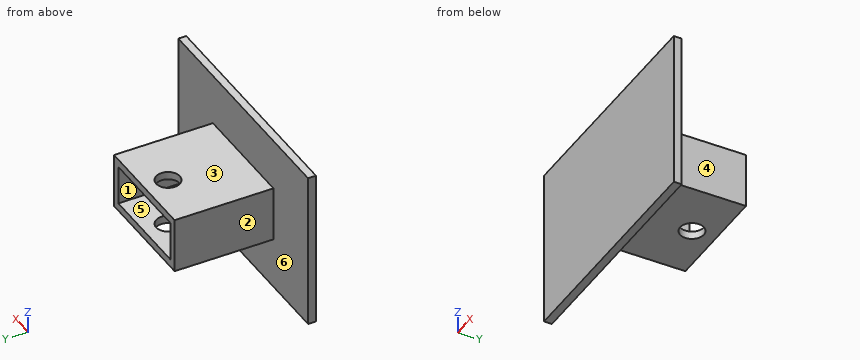
```python
from build123d import *

# Parameters (mm, degrees)
SKETCH1_W           = 76.2
SKETCH1_H           = 50.8
BOSS_EXTRUDE1_DEPTH = 2.54
SKETCH2_W           = 35.56
SKETCH2_H           = 17.78
SKETCH2_W_2         = 30.48
SKETCH2_H_2         = 12.7
BOSS_EXTRUDE2_DEPTH = 31.75
SKETCH3_R           = 3.81
CUT_EXTRUDE1_DEPTH  = 31.75


with BuildPart() as part:
    # Sketch1 → Boss-Extrude1 (new body)
    with BuildSketch(Plane(origin=(0, 0, 0), x_dir=(1, 0, 0), z_dir=(0, 1, 0))):
        Rectangle(SKETCH1_W, SKETCH1_H)
    extrude(amount=BOSS_EXTRUDE1_DEPTH)

    # Sketch2 → Boss-Extrude2 (add)
    with BuildSketch(Plane(origin=(0, 2.54, 0), x_dir=(1, 0, 0), z_dir=(0, 1, 0))):
        Rectangle(SKETCH2_W, SKETCH2_H)
        Rectangle(SKETCH2_W_2, SKETCH2_H_2, mode=Mode.SUBTRACT)
    extrude(amount=BOSS_EXTRUDE2_DEPTH)

    # Sketch3 → Cut-Extrude1 (cut)
    with BuildSketch(Plane.XY.offset(8.89)):
        with Locations((0, 26.67)):
            Circle(SKETCH3_R)
    extrude(amount=-CUT_EXTRUDE1_DEPTH, mode=Mode.SUBTRACT)


solid = part.part
```
For this review, take the finished solid that the model builds, in its own axes (mm). Face numbers are marked on the shaded views. A direction names the side the tool comes from. Give positions to 0.01 mm unless a question says otherwise; leave off trailing zeros. Write each loop counter-clockwise with the first axis right and the second up, starting at its lowest first coordinate (ties: lowest second). Pieces come first, ordered by that corner, then holes.
Item 1: Take a section at C-C (z = -1.5). Give the boundary of the cut face in (x, y), and give its area (3 significant figures).
Item 2: Wall thickness on probe 1 along Z at (x, y) = (-12, 22.5); probe 2 along X at (y, z) = (5, 5.5); probe 3 along Y at (x, z) = (0, 7.3): over which ranges is each line inside the solid? List them lowest first.
Item 3: Take a section at A-A (x = 0). Give the boundary of the cut face in (y, z).
Item 4: Insertion check: P1, Ø1.5, axis at x = 14.5, y = 16, coming from the -Z side; P2, Ø19.5, axis at y = 12.5, z = -0.5, coming from the -X side; P3, Ø10, axis at y = 21.5, z = -2, coming from the +X side. Each pin has a flat end and moves straight along its axis. Give the tip position at first contact, or say it passes through.
Item 5: Take a section at B-B (y = 26.67). Give the boundary of the cut face in (x, z).
Item 6: Take a section at D-D (x = -16.5). Give the boundary of the cut face in (y, z).
Item 7: Machinability: for the marked faces 1, 2 and 3, which of the approach directions +Z, -Z, +X, -X, +Y, -Y give a long, thin tool a straight path to every point of the face, cutting with its end or side? Answer none if there is none.
Item 8: The part is to be moulded in two halves that separate along X. For the marked faces 4, 5 and 6, say which applies: +X half, -X half, draft (parallel to the pull), parting line (faces both ways), or undercut.
Established:
1. outline: (-38.1, 0) - (38.1, 0) - (38.1, 2.54) - (17.78, 2.54) - (17.78, 34.29) - (15.24, 34.29) - (15.24, 2.54) - (-15.24, 2.54) - (-15.24, 34.29) - (-17.78, 34.29) - (-17.78, 2.54) - (-38.1, 2.54) - close
1. area: 355 mm2
2. probe 1: z = -8.89 to -6.35, 6.35 to 8.89
2. probe 2: x = -17.78 to -15.24, 15.24 to 17.78
2. probe 3: y = 0 to 22.86, 30.48 to 34.29
3. outline: (0, -25.4) - (2.54, -25.4) - (2.54, -8.89) - (22.86, -8.89) - (22.86, -6.35) - (2.54, -6.35) - (2.54, 6.35) - (22.86, 6.35) - (22.86, 8.89) - (2.54, 8.89) - (2.54, 25.4) - (0, 25.4) - close; (30.48, -8.89) - (34.29, -8.89) - (34.29, -6.35) - (30.48, -6.35) - close; (30.48, 6.35) - (34.29, 6.35) - (34.29, 8.89) - (30.48, 8.89) - close
4. P1: stops at z = -8.89
4. P2: stops at x = -17.78
4. P3: stops at x = 17.78
5. outline: (-17.78, -8.89) - (-3.81, -8.89) - (-3.81, -6.35) - (-15.24, -6.35) - (-15.24, 6.35) - (-3.81, 6.35) - (-3.81, 8.89) - (-17.78, 8.89) - close; (3.81, -8.89) - (17.78, -8.89) - (17.78, 8.89) - (3.81, 8.89) - (3.81, 6.35) - (15.24, 6.35) - (15.24, -6.35) - (3.81, -6.35) - close
6. outline: (0, -25.4) - (2.54, -25.4) - (2.54, -8.89) - (34.29, -8.89) - (34.29, 8.89) - (2.54, 8.89) - (2.54, 25.4) - (0, 25.4) - close
7. face 1: +Y
7. face 2: +Z, -Z, -X, +Y
7. face 3: +Z, +X, -X, +Y
8. face 4: +X half
8. face 5: undercut
8. face 6: draft
